Could you check a few things on this drawing? It's one solid part, dimensions in mm from its lowest x, y, z. Give positions to 0.01 mm unless a question says otherwise; leave off trailing zeros. Order: outer loops, then holes, each group sorted by start corner. A loop starts at its lowest first (then second) coordinate and runs counter-clockwise, first axis right, second up. Notation, with made-up numbers: (85, 23) - (138, 23) arc R19 ccw to (138, 56) - close; hole circle Ø1 at (15.25, -26). An arc over 180 degrees is marked (long way). Put each result on its own line as item: value.
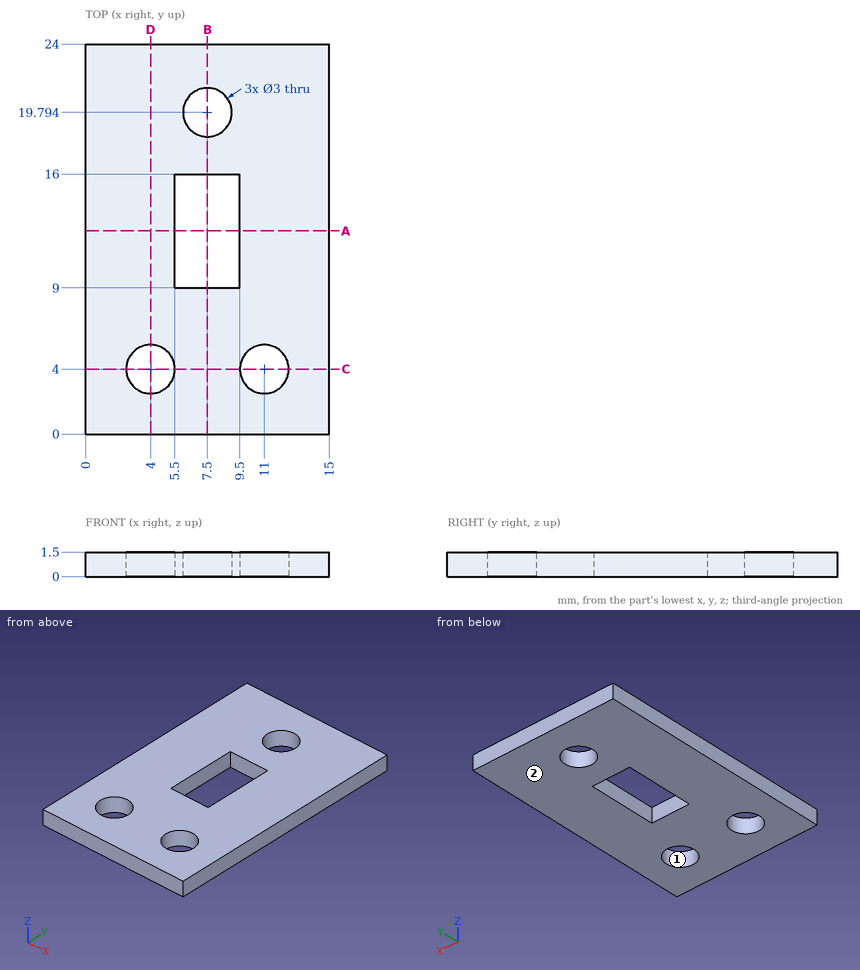
1) Suppose I cut it at C-C, the plane y = 4. List the corners of the cut face in (x, z) for me.
Filled in:
outline: (0, 0) - (2.5, 0) - (2.5, 1.5) - (0, 1.5) - close; (5.5, 0) - (9.5, 0) - (9.5, 1.5) - (5.5, 1.5) - close; (12.5, 0) - (15, 0) - (15, 1.5) - (12.5, 1.5) - close
2) Suppose I cut it at A-A, the plane y = 12.5. List the corners of the cut face in (x, z) for me.
Filled in:
outline: (0, 0) - (5.5, 0) - (5.5, 1.5) - (0, 1.5) - close; (9.5, 0) - (15, 0) - (15, 1.5) - (9.5, 1.5) - close
3) We'd pull the mould along X, two halves only. Please class the marked faces 1 and 2: pulls with the +X half, pulls with the -X half, needs draft (parallel to the pull), parting line crosses it, or undercut.
Filled in:
face 1: undercut
face 2: needs draft
4) If I drill on line 1 (Y direction, x = 11, z = 1.05); line 2 (Y direction, x = 7.5, z = 0.85); line 3 (Y direction, x = 8, z = 0.25), over which ranges is the centre line in solid material (lowest first)? Write a range as [from, to].
Filled in:
line 1: y = [0, 2.5], [5.5, 24]
line 2: y = [0, 9], [16, 18.29], [21.29, 24]
line 3: y = [0, 9], [16, 18.38], [21.21, 24]
5) Suppose I cut it at D-D, the plane x = 4. List the corners of the cut face in (y, z) for me.
Filled in:
outline: (0, 0) - (2.5, 0) - (2.5, 1.5) - (0, 1.5) - close; (5.5, 0) - (24, 0) - (24, 1.5) - (5.5, 1.5) - close
6) I'm going to push flat-ended pins straight in: pin 1 (2.5 mm diameter, centred on x = 11, y = 4, fed in from +Z); pin 2 (5 mm diameter, centred on x = 7.5, y = 19.79, fed in from -Z). Where does each tip first touch, or does it pass through?
Filled in:
pin 1: passes through
pin 2: stops at z = 0
7) Suppose I cut it at B-B, the plane x = 7.5. List the corners of the cut face in (y, z) for me, and give its area (3 significant figures).
Filled in:
outline: (0, 0) - (9, 0) - (9, 1.5) - (0, 1.5) - close; (16, 0) - (18.29, 0) - (18.29, 1.5) - (16, 1.5) - close; (21.29, 0) - (24, 0) - (24, 1.5) - (21.29, 1.5) - close
area: 21.0 mm^2
